from build123d import *

# Parameters (mm, degrees)
CROQUIS1_R                   = 40
SALIENTE_EXTRUIR1_DEPTH      = 15
CORTAR_EXTRUIR3_START        = -55
CORTAR_EXTRUIR3_DEPTH        = 75
MATRIZC1_COUNT               = 38
SALIENTE_EXTRUIR2_DEPTH      = 18
SALIENTE_EXTRUIR2_DEPTH_BACK = 3
CROQUIS4_R                   = 12.5
CROQUIS4_R_2                 = 10
CORTAR_EXTRUIR4_DEPTH        = 26
CORTAR_EXTRUIR4_DEPTH_BACK   = 41
CROQUIS5_R                   = 2.5


with BuildPart() as part:
    # Croquis1 → Saliente-Extruir1 (new body)
    with BuildSketch(Plane(origin=(0, 0, 0), x_dir=(1, 0, 0), z_dir=(0, 1, 0))):
        with Locations(Location((0, 0, 0), (0, 0, 270))):
            Circle(CROQUIS1_R)
    extrude(amount=SALIENTE_EXTRUIR1_DEPTH)

    # Croquis2 → Cortar-Extruir3 (cut)
    with BuildSketch(Plane(origin=(0, 0, 0), x_dir=(1, 0, 0), z_dir=(0, 1, 0)).offset(CORTAR_EXTRUIR3_START)):
        Polygon((0, 34.025968572), (3.276888375, 39.865549069), (0, 41.704379346), (-3.276888375, 39.865549069), align=None)
    cortar_extruir3 = extrude(amount=CORTAR_EXTRUIR3_DEPTH, mode=Mode.SUBTRACT)

    # MatrizC1: Cortar-Extruir3 ×38 about axis
    matrizc1_axis = Axis((0, 0, 0), (0, 1, 0))
    for i in range(1, MATRIZC1_COUNT):
        add(cortar_extruir3.rotate(matrizc1_axis, i * 360 / MATRIZC1_COUNT), mode=Mode.SUBTRACT)

    # Croquis4 → Saliente-Extruir2 (add, two sides: drawn at the far end of the back side and taken through both)
    with BuildSketch(Plane(origin=(0, 0, 0), x_dir=(1, 0, 0), z_dir=(0, 1, 0)).offset(-SALIENTE_EXTRUIR2_DEPTH_BACK)):
        with Locations(Location((0, 0, 0), (0, 0, 270))):
            Circle(CROQUIS4_R)
        with Locations(Location((0, 0, 0), (0, 0, 270))):
            Circle(CROQUIS4_R_2, mode=Mode.SUBTRACT)
    extrude(amount=SALIENTE_EXTRUIR2_DEPTH + SALIENTE_EXTRUIR2_DEPTH_BACK)

    # Croquis5 → Cortar-Extruir4 (cut, two sides: drawn at the far end of the back side and taken through both)
    with BuildSketch(Plane(origin=(0, 0, 0), x_dir=(1, 0, 0), z_dir=(0, 1, 0)).offset(-CORTAR_EXTRUIR4_DEPTH_BACK)):
        with Locations(Location((0, 0, 0), (0, 0, 270))):
            Circle(CROQUIS5_R)
    extrude(amount=CORTAR_EXTRUIR4_DEPTH + CORTAR_EXTRUIR4_DEPTH_BACK, mode=Mode.SUBTRACT)


solid = part.part
Here's how the part is built. I have some questions about the finished solid (model axes, mm). A direction names the side the tool comes from. Give positions to 0.01 mm unless a question says otherwise; leave off trailing zeros. Answer as a JSON object with one key per item and string values. Group by question number.
Item 1: On a 3-axis mill with a long thin cutter (end or side, diameter ignored), from which of +Z, -Z, +X, -X, +Y, -Y can I reach the whole of each face in a straight line? I mean faces 1 (the flat face through (-31.87, 7.39, -18.84)), 2 (the flat face through (9, 0, -9)), 3 (the flat face through (-36.26, 7.39, -7.47)). Say none if no direction works.
Item 2: I need wall thicknesses on L1, parallel to X at y = -1.2, z = 0; L2, parallel to X at y = 3.5, z = -34.5. Which ranges of each line are inside material? Lowest first, please.
Item 3: Will these pins go through, and if not, where does the flat tip stop? pin 1 (16 mm diameter, centred on x = 0, z = 0, fed in from -Y); pin 2 (1 mm diameter, centred on x = 30.5, y = 5, fed in from -Z); pin 3 (8 mm diameter, centred on x = 31, y = 0.5, fed in from -Z).
Item 4: Thinking about a two-plate mould opening in X: for faces 4 (the flat face through (34.445, 7.395, -13.345)), 5 (the flat face through (23.94, 7.39, -28.13)), 6 (the flat face through (-36.91, 7.39, 1.44)), which applies, pulls with the +X half, pulls with the -X half, needs draft (parallel to the pull), parting line crosses it, or undercut?
Answer list:
{
 "1": {"face 1": "+Y, -Y", "face 2": "-Y", "face 3": "-X, +Y, -Y"},
 "2": {"L1": "x = -12.5 to -10, 10 to 12.5", "L2": "x = -16.12 to -13.64, -10.62 to -6.35, -5.26 to -0.27, 0.27 to 5.26, 6.35 to 10.62, 13.64 to 16.12"},
 "3": {"pin 1": "stops at y = 0", "pin 2": "stops at z = -24.46", "pin 3": "stops at z = -29.45"},
 "4": {"face 4": "pulls with the +X half", "face 5": "undercut", "face 6": "pulls with the -X half"}
}
